Check sheet for the modelled part. Datum: model origin and axes. Units: mm. Face numbers are marked on the shaded views. A direction names the side the tool comes from. Give positions to 0.01 mm unless a question says otherwise; leave off trailing zeros. Write each loop counter-clockwise with the first axis right and the second up, starting at its lowest first coordinate (ties: lowest second). Pieces come first, ordered by that corner, then holes. Notation, with made-up numbers: M 3.25,83 L 21.25,83 A35 ccw 21.25,115 Z; hole C 53,-16.75 d6. An arc over 180 degrees is marked long. One line per item, written item: value. Start each with the question number.
from build123d import *

# Parameters (mm, degrees)
SKETCH1_W           = 1200
SKETCH1_H           = 620
BOSS_EXTRUDE1_DEPTH = 12
SKETCH2_W           = 12
SKETCH2_H           = 174.6
BOSS_EXTRUDE2_DEPTH = 80
SKETCH6_W           = 1200
SKETCH6_H           = 174.6
BOSS_EXTRUDE5_DEPTH = 12
SKETCH7_W           = 305
SKETCH7_H           = 12
BOSS_EXTRUDE6_DEPTH = 230
SKETCH8_W           = 539.2
SKETCH8_H           = 35
BOSS_EXTRUDE7_DEPTH = 12


with BuildPart() as part:
    # Sketch1 → Boss-Extrude1 (new body)
    with BuildSketch(Plane(origin=(0, 0, 0), x_dir=(1, 0, 0), z_dir=(0, 1, 0))):
        Rectangle(SKETCH1_W, SKETCH1_H)
    extrude(amount=BOSS_EXTRUDE1_DEPTH)

    # Sketch2 → Boss-Extrude2 (add)
    with BuildSketch(Plane(origin=(0, 12, 0), x_dir=(1, 0, 0), z_dir=(0, 1, 0))):
        with Locations((-594, 197.3)):
            Rectangle(SKETCH2_W, SKETCH2_H)
        with Locations((-104, 197.3)):
            Rectangle(SKETCH2_W, SKETCH2_H)
        with Locations((104, 197.3)):
            Rectangle(SKETCH2_W, SKETCH2_H)
        with Locations((594, 197.3)):
            Rectangle(SKETCH2_W, SKETCH2_H)
    extrude(amount=BOSS_EXTRUDE2_DEPTH)

    # Sketch6 → Boss-Extrude5 (add)
    with BuildSketch(Plane(origin=(0, 92, 0), x_dir=(1, 0, 0), z_dir=(0, 1, 0))):
        with Locations((0, 197.3)):
            Rectangle(SKETCH6_W, SKETCH6_H)
    extrude(amount=BOSS_EXTRUDE5_DEPTH)

    # Sketch7 → Boss-Extrude6 (add)
    with BuildSketch(Plane(origin=(0, 12, 0), x_dir=(1, 0, 0), z_dir=(0, 1, 0))):
        with Locations((-447.5, 290.6)):
            Rectangle(SKETCH7_W, SKETCH7_H)
        with Locations((447.5, 290.6)):
            Rectangle(SKETCH7_W, SKETCH7_H)
    extrude(amount=BOSS_EXTRUDE6_DEPTH)

    # Sketch8 → Boss-Extrude7 (add)
    with BuildSketch(Plane(origin=(0, 0, -284.6), x_dir=(-1, 0, 0), z_dir=(0, 0, -1))):
        with Locations((0, 86.5)):
            Rectangle(SKETCH8_W, SKETCH8_H)
    extrude(amount=BOSS_EXTRUDE7_DEPTH)


solid = part.part
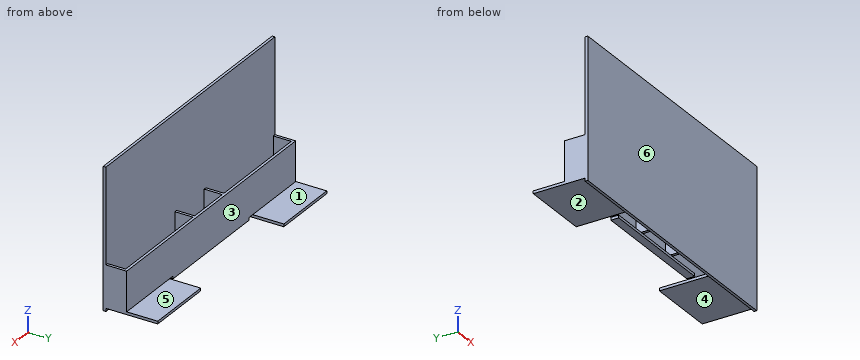
1) Cross-section at D-D (x = 400). Record the boundary of the cut face in (y, z), plus the area to 3 significant figures.
2) Cross-section at C-C (z = -122.5). Record the boundary of the cut face in (x, y).
3) Tool access check on the marked faces 4, 5 and 6. Record the directions out of +Z, -Z, +X, -X, +Y, -Y that give a thin tool (end or side, any length) a straight path to the whole face; none if there is none.
4) Draft check along Z on the marked faces 1, 2 and 3. Enter one of: released by +Z, released by -Z, zero draft, split by the parting line, or undercut.
5) Cross-section at B-B (y = 132). Record the boundary of the cut face in (x, z).
6) Material ranges on L1, parallel to X at y = 34, z = -259.5; L2, parallel to Y at x = -210, z = -151; L3, parallel to Y at x = -254.5, z = -53, recorded low to high. Write a range as from..to.
7) Gauge pin test, flat ends, axial feed: pin 1 (9.5 mm diameter, centred on x = 101, y = 52, fed in from -Z); pin 2 (1 mm diameter, centred on x = 76.5, z = 112, fed in from +Y); pin 3 (4 mm diameter, centred on x = 359.5, z = -220, fed in from +Y). Record the tip position at first contact, or that the pin passes through.
8) Cross-section at A-A (x = 223). Record the boundary of the cut face in (y, z), plus the area to 3 significant figures.
Data:
1. outline: M 0,-310 L 12,-310 L 12,-296.6 L 242,-296.6 L 242,-284.6 L 104,-284.6 L 104,-110 L 92,-110 L 92,-284.6 L 12,-284.6 L 12,310 L 0,310 Z
1. area: 12,300 mm2
2. outline: M -600,0 L 600,0 L 600,104 L -600,104 Z; hole M -588,12 L -110,12 L -110,92 L -588,92 Z; hole M -98,12 L 98,12 L 98,92 L -98,92 Z; hole M 110,12 L 588,12 L 588,92 L 110,92 Z
3. face 4: -Z, +X, -X, +Y
3. face 5: +Z, +X, -X, +Y
3. face 6: +Z, -Z, +X, -X, -Y
4. face 1: released by +Z
4. face 2: released by -Z
4. face 3: zero draft
5. outline: M -600,-296.6 L -295,-296.6 L -295,-284.6 L -600,-284.6 Z; M 295,-296.6 L 600,-296.6 L 600,-284.6 L 295,-284.6 Z
6. L1: x = -600..-588, -110..-98, 98..110, 588..600
6. L2: y = 0..12, 92..104
6. L3: y = 0..12
7. pin 1: stops at z = -284.6
7. pin 2: stops at y = 12
7. pin 3: stops at y = 104
8. outline: M 0,-310 L 12,-310 L 12,310 L 0,310 Z; M 69,-296.6 L 104,-296.6 L 104,-110 L 92,-110 L 92,-284.6 L 69,-284.6 Z
8. area: 9,960 mm2
